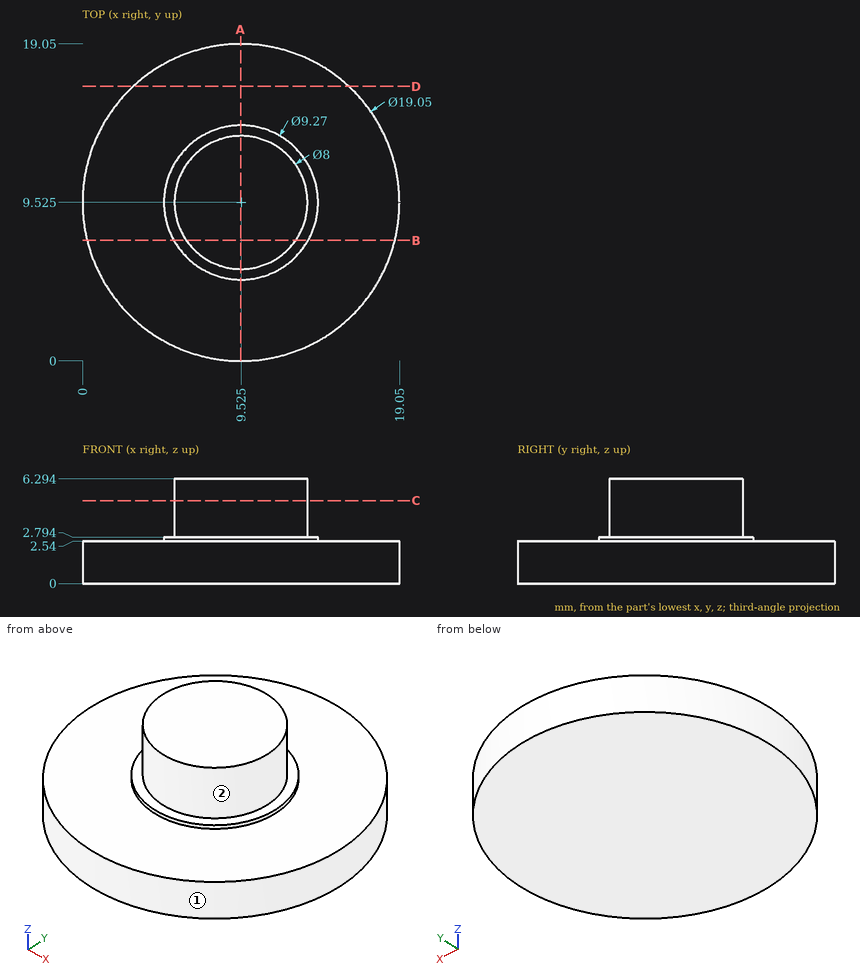
Design review of the part shown in the three views and the two pictorial views. Dimensions are in mm from the part's minimum x, y and z. A direction names the side the tool comes from. Give positions to 0.01 mm unless a question says otherwise; leave off trailing zeros. Loops run counter-clockwise (first coordinate to the right, second up) from the corner with the lowest first, then second, coordinate; pieces in that order, holes last. Notation, with made-up numbers: (-15.75, -25.5) - (3.25, -25.5) arc R22 cw to (3.25, -0.5) - close; hole circle Ø10 at (54, 8). An arc over 180 degrees is marked (long way). Answer as a JSON object with one key per item and string values.
Q1. Add section B-B on y = 7.25. State the section outline as (x, z) points, plus the area to 3 significant figures.
Worked out:
{"outline": "(0.28, 0) - (18.77, 0) - (18.77, 2.54) - (13.56, 2.54) - (13.56, 2.79) - (12.82, 2.79) - (12.82, 6.29) - (6.23, 6.29) - (6.23, 2.79) - (5.49, 2.79) - (5.49, 2.54) - (0.28, 2.54) - close", "area": "72.1 mm^2"}
Q2. Add section C-C on z = 5. State the section outline as (x, y) points (3 decimals), plus the area to 3 significant figures.
Worked out:
{"outline": "circle Ø8 at (9.525, 9.525)", "area": "50.3 mm^2"}
Q3. Add section A-A on x = 9.5. State the section outline as (y, z) points, plus the area to 3 significant figures.
Worked out:
{"outline": "(0, 0) - (19.05, 0) - (19.05, 2.54) - (14.16, 2.54) - (14.16, 2.79) - (13.52, 2.79) - (13.52, 6.29) - (5.53, 6.29) - (5.53, 2.79) - (4.89, 2.79) - (4.89, 2.54) - (0, 2.54) - close", "area": "78.7 mm^2"}
Q4. Add section D-D on y = 16.5. State the section outline as (x, z) points, plus the area to 3 significant figures.
Worked out:
{"outline": "(3.04, 0) - (16.01, 0) - (16.01, 2.54) - (3.04, 2.54) - close", "area": "33.0 mm^2"}
Q5. To check wall thickness, follow line 1 along Z through (x, y) = (15, 7); line 2 along Z through (x, y) = (10.5, 13.5); line 3 along X through (y, z) = (15.75, 0.5). State the ranges of each line that lie inside material, in increasing order.
Worked out:
{"line 1": "z = 0 to 2.54", "line 2": "z = 0 to 2.79", "line 3": "x = 2.32 to 16.73"}
Q6. For the marked faces 1 and 2, list the 3-axis set-ups (+Z, -Z, +X, -X, +Y, -Y) from which the entire face can be reached by the end or side of a thin tool; tool diameter is ignored.
Worked out:
{"face 1": "+Z, -Z", "face 2": "+Z"}
Q7. Insertion check: pin 1 (2 mm diameter, centred on y = 5.5, z = 2.5, fed in from -X). The pin has a flat end and moves straight along its axis. Give the tip position at first contact, or say it passes through.
Worked out:
{"pin 1": "stops at x = 0.49"}
